Autodesk Fusion 360 part; units mm, degrees
sketch "Sketch1" plane through (0, 0, 0) normal (0, 0, 1) x (1, 0, 0)
  line L0 (-15, -11) -> (15, -11)
  line L1 (15, -11) -> (15, 11)
  line L2 (15, 11) -> (-15, 11)
  line L3 (-15, 11) -> (-15, -11)
  line L4 (-15, -11) -> (15, 11) construction
  line L5 (15, -11) -> (-15, 11) construction
  circle A0 centre (32, 0) radius 8
  line L6 (0, 0) -> (32, 0) construction
  line L7 (85, -15) -> (-25, -15)
  line L8 (-25, -15) -> (-25, 15)
  line L9 (-25, 15) -> (85, 15)
  line L10 (85, 15) -> (85, -15)
  line L11 (85, -15) -> (-25, 15) construction
  line L12 (-25, -15) -> (85, 15) construction
  line L13 (83, -13) -> (-23, -13)
  line L14 (-23, -13) -> (-23, 13)
  line L15 (-23, 13) -> (83, 13)
  line L16 (83, 13) -> (83, -13)
  line L17 (74, -7.5) -> (50, -7.5)
  line L18 (50, -7.5) -> (50, 7.5)
  line L19 (50, 7.5) -> (74, 7.5)
  line L20 (74, 7.5) -> (74, -7.5)
  line L21 (74, -7.5) -> (50, 7.5) construction
  line L22 (50, -7.5) -> (74, 7.5) construction
  line L23 (24, 13) -> (24, -13) construction
  line L24 (40, 13) -> (40, -13) construction
  line L25 (32, 0) -> (62, 0) construction
  point P0 (30, 0)
  point P1 (62, 0)
  dimension "d1" = 30
  dimension "d2" = 22
  dimension "d3" = 16
  dimension "d5" = 30
  dimension "d6" = 10
  dimension "d7" = 2
  dimension "d12" = 24
  dimension "d13" = 15
  dimension "d14" = 9
  dimension "d15" = 10
  dimension "d16" = 9
  dimension "d30" = 110
extrude "Extrude2" add sketch "Sketch1" against normal blind 4 contours L7 L8 L9 L10 | L13 L14 L15 L16 makes body 1
extrude "Extrude3" add sketch "Sketch1" against normal blind 42 contours L7 L8 L9 L10 bodies 1
extrude "Extrude4" add sketch "Sketch1" against normal blind 26.4 separate body contours L0 L1 L2 L3 makes body 2
sketch "Sketch4" plane through (-25, 0, 0) normal (-1, 0, 0) x (0, -1, 0)
  line L0 (15, 0) -> (-15, 0)
  line L1 (-15, 0) -> (-15, -42)
  line L2 (-15, -42) -> (15, -42)
  line L3 (15, -42) -> (15, 0)
  line L4 (-15, -42) -> (15, -24.6795)
  dimension "d24" = 60
extrude "Extrude5" cut sketch "Sketch4" against normal through all contours L2 L3 L4 bodies 1 2
sketch "Sketch5" plane through (0, -14.4365, -25.0048) normal (0, -0.5, -0.866) x (1, 0, 0)
  line L0 (-23, -1.6588) -> (83, -1.6588)
  line L1 (83, -1.6588) -> (83, -31.681)
  line L2 (83, -31.681) -> (-23, -31.681)
  line L3 (-23, -31.681) -> (-23, -1.6588)
  line L4 (85, -33.9904) -> (85, 0.6506)
  line L5 (85, 0.6506) -> (-25, 0.6506)
  line L6 (-25, 0.6506) -> (-25, -33.9904)
  line L7 (-25, -33.9904) -> (85, -33.9904)
  line L8 (-25, -11.5312) -> (85, -11.5312) construction
  circle A0 centre (-20, -11.5312) radius 1.5
  circle A1 centre (80, -11.5312) radius 1.5
  circle A2 centre (-20, -11.5312) radius 4
  circle A3 centre (80, -11.5312) radius 4
  line L9 (-25, -7.5312) -> (-20, -7.5312)
  line L10 (-25, -15.5312) -> (-20, -15.5312)
  line L11 (85, -7.5312) -> (80, -7.5312)
  line L12 (85, -15.5312) -> (80, -15.5312)
  dimension "d26" = 3
  dimension "d27" = 3
  dimension "d28" = 100
  dimension "d29" = 5
  dimension "d31" = 5
  dimension "d32" = 8
  dimension "d33" = 8
extrude "Extrude6" add sketch "Sketch5" against normal blind 31.9 contours L3 A2 L9 | L1 A3 L11 | L3 A2 | L1 A3 | L3 A2 L10 | L1 A3 L12 picked at (-22.5, -11.5312) picked at (82.5, -11.5312) bodies 1
fillet "Fillet3" radius 5 4 edges at (83, 13, -24.6955) (83, -13, -14.9171) (-23, 13, -24.6955) (-23, -13, -14.9171) on bodies 1
fillet "Fillet1" radius 2 2 edges at (30, -13, -4) (30, 13, -4) on bodies 1
sketch "Sketch6" plane through (0, 15, 0) normal (0, 1, 0) x (-1, 0, 0)
  line L0 (25, 0) -> (-85, 0)
  line L1 (-85, 0) -> (-85, -42)
  line L2 (-85, -42) -> (25, -42)
  line L3 (25, -42) -> (25, 0)
  circle A0 centre (-65, -42) radius 7.5
  circle A1 centre (-30, -42) radius 7.5
  circle A2 centre (5, -42) radius 7.5
  dimension "d39" = 15
  dimension "d40" = 15
  dimension "d41" = 15
  dimension "d42" = 20
  dimension "d43" = 20
extrude "Extrude8" cut sketch "Sketch6" against normal blind 5 contours L2 A2 | L2 A0 | L2 A1 picked at (5.1868, -39.507) picked at (-65.5284, -39.1901) picked at (-29.8132, -39.507) bodies 1
fillet "Fillet2" radius 5 4 edges at (-25, -15, -12.3397) (-25, 15, -21) (85, -15, -12.3397) (85, 15, -21) on bodies 1
hidden bodies 2
Geometry check sheet. Reference: the model listing, model coordinates, mm. A direction names the side the tool comes from. Give positions to 0.01 mm unless a question says otherwise; leave off trailing zeros. Loops run counter-clockwise (first coordinate to the right, second up) from the corner with the lowest first, then second, coordinate; pieces in that order, holes last. Notation, with made-up numbers: (9.25, 64) -> (23.25, 64) arc R12 cw to (23.25, 76) -> close; hole circle Ø5 at (10.25, 17). An arc over 180 degrees is marked (long way). Answer in a Markdown table with one row per item. Add a question column.
1) Cross-section at C-C on y = 0. State how many separate pieces and enclosed holes the cut face has, and give its area (3 significant figures).
2) Cross-section at B-B on x = 65. Record the boundary of the cut face in (y, z).
3) Material ranges on probe 1 along Y at (x, z) = (-13.5, -15.5); probe 2 along Y at (x, z) = (32, -3.1); probe 3 along Y at (x, z) = (79, -13), recorded low to high. Write a range as from..to.
4) Gauge pin test, flat ends, axial feed: P1, Ø1.5, axis at x = 51.5, y = 8, coming from the -Z side; P2, Ø0.9, axis at x = -20.5, y = 11.5, coming from the -Z side. Record the tip position at first contact, or that the pin passes through.
5) Set-up check for faces 5 (the face through (-21.521, -0.864, -16.559)), 6 (the face through (-25, 0, -15)), 7 (the face through (74, 0, -2)), 8 (the face through (-23, -14, -14)), 9 (the face through (-21, -12, -18)): record each of +Z, -Z, +X, -X, +Y, -Y from which the full face is reachable in a straight line by a thin tool's end or side.
6) Draft check along Z on faces 1 (the face through (83, -3, -15)), 2 (the face through (47.36, 14.01, -41.43)), 3 (the face through (80, 11, -4)), 4 (the face through (31, -13, -16)). Enter one of: pulls with the +Z half, pulls with the -Z half, needs draft (parallel to the pull), parting line crosses it, or undercut.
Outcome:
| question | item | result |
|---|---|---|
| 1 | separate pieces | 4 |
| 1 | enclosed holes | 2 |
| 1 | area | 447 mm^2 |
| 2 | outline | (-15, -24.68) -> (-13, -25.83) -> (-13, -6) arc R2 cw to (-11, -4) -> (-7.5, -4) -> (-7.5, 0) -> (-15, 0) -> close; (7.5, -4) -> (11, -4) arc R2 cw to (13, -6) -> (13, -34.5) -> (15, -34.5) -> (15, 0) -> (7.5, 0) -> close |
| 3 | probe 1 | y = -15..-13, 13..15 |
| 3 | probe 2 | y = -15..-8, 8..15 |
| 3 | probe 3 | y = -15..-12.9, 1.34..4.52, 7.1..10.28, 12.9..15 |
| 4 | P1 | stops at z = -4 |
| 4 | P2 | stops at z = -11.92 |
| 5 | face 5 | none |
| 5 | face 6 | +Z, -Z, -X, +Y, -Y |
| 5 | face 7 | +Z, -Z |
| 5 | face 8 | +Z, -Z, -X, -Y |
| 5 | face 9 | -Z |
| 6 | face 1 | undercut |
| 6 | face 2 | pulls with the -Z half |
| 6 | face 3 | undercut |
| 6 | face 4 | needs draft |
